Could you check a few things on this drawing? It's one solid part, dimensions in mm from its lowest x, y, z. A direction names the side the tool comes from. Give positions to 0.01 mm unless a question says otherwise; leave off trailing zeros. Loops run counter-clockwise (first coordinate to the right, second up) from the corner with the lowest first, then second, coordinate; pieces in that order, holes last. Notation, with made-up numbers: M 25.5,61 L 70.5,61 A38 ccw 70.5,99 Z; hole C 74,87.5 d9. An arc over 180 degrees is marked long. One line per item, written item: value. Start each with the question number.
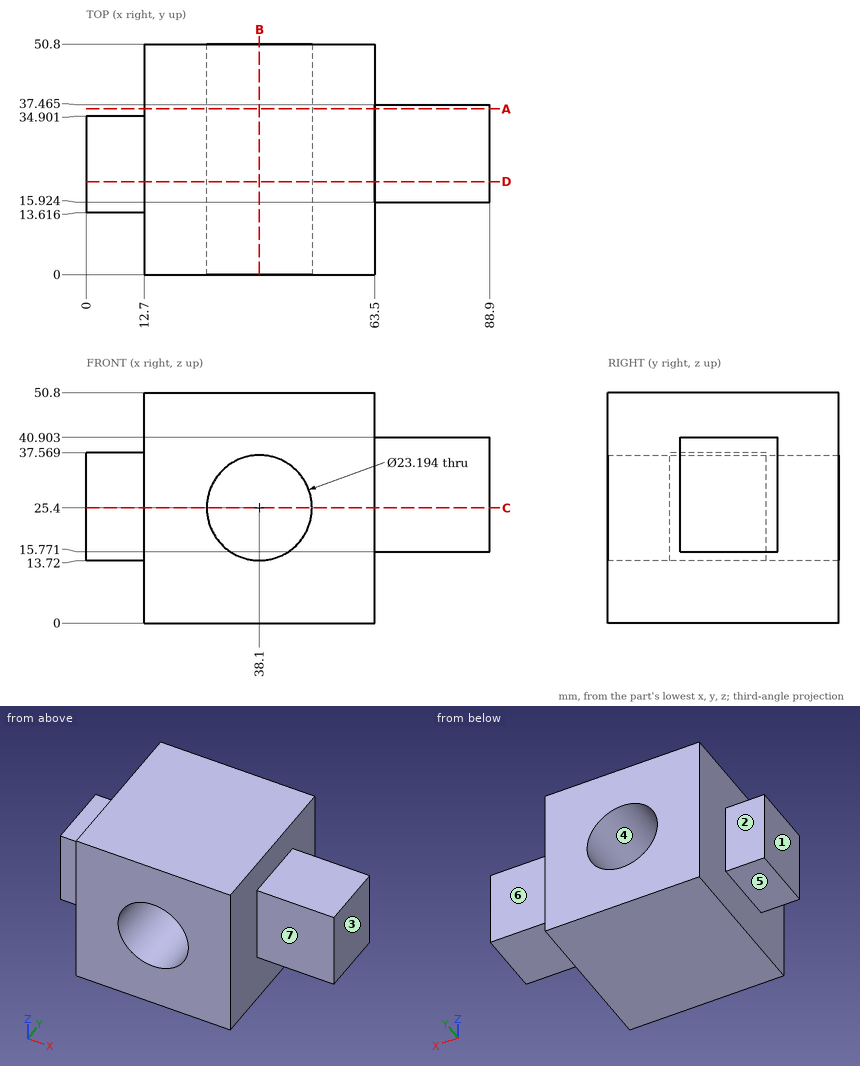
Q1. If we section it at A-A, the plane y = 36.5: Write out the boundary of the cut face in (x, z).
Q2. If we mould it in two halves opening along X, with no side actions, what happens to the marked faces 1, 2, 3 and 4? For each: released by +X, released by -X, zero draft, split by the parting line, or undercut.
Q3. Which directions (+Z, -Z, +X, -X, +Y, -Y) give clear straight access to the entire face, cutting with the end or side of a thin tool? Please do the marked faces 5, 6 and 7.
Q4. If we section it at B-B, the plane x = 38.1: Write out the boundary of the cut face in (y, z).
Q5. For P1, Ø4, axis at y = 23.5, z = 23.5, coming from the -X side; P2, Ø1, axis at y = 35.5, z = 16.5, coming from the -X side; P3, Ø6.5, axis at x = 70, y = 28.5, coming from the -Z side; P4, Ø6.5, axis at x = 8, z = 21, coming from the +Y side, each with a flat end and sliding along its axis, tell me the tip position at first contact or that it passes through.
Q6. If we section it at C-C, the plane z = 25.4: Write out the boundary of the cut face in (x, y) (1 decimal).
Q7. I need wall thicknesses on line 1 along Z through (x, y) = (38, 14); line 2 along X through (y, z) = (15, 25); line 3 along X through (y, z) = (29, 8). Which ranges of each line are inside material? Lowest first, please.
Q8. If we section it at D-D, the plane y = 20.5: Write out the boundary of the cut face in (x, z).
Response:
1. outline: M 12.7,0 L 63.5,0 L 63.5,15.77 L 88.9,15.77 L 88.9,40.9 L 63.5,40.9 L 63.5,50.8 L 12.7,50.8 Z; hole C 38.1,25.4 d23.19
2. face 1: released by -X
2. face 2: zero draft
2. face 3: released by +X
2. face 4: undercut
3. face 5: -Z, -X, +Y, -Y
3. face 6: +Z, -Z, +X, +Y
3. face 7: +Z, -Z, +X, -Y
4. outline: M 0,0 L 50.8,0 L 50.8,13.8 L 0,13.8 Z; M 0,37 L 50.8,37 L 50.8,50.8 L 0,50.8 Z
5. P1: x = 0
5. P2: x = 12.7
5. P3: z = 15.77
5. P4: y = 34.9
6. outline: M 0,13.6 L 12.7,13.6 L 12.7,0 L 26.5,0 L 26.5,50.8 L 12.7,50.8 L 12.7,34.9 L 0,34.9 Z; M 49.7,0 L 63.5,0 L 63.5,15.9 L 88.9,15.9 L 88.9,37.5 L 63.5,37.5 L 63.5,50.8 L 49.7,50.8 Z
7. line 1: 0 to 13.8, 37 to 50.8
7. line 2: 0 to 26.51, 49.69 to 63.5
7. line 3: 12.7 to 63.5
8. outline: M 0,13.72 L 12.7,13.72 L 12.7,0 L 63.5,0 L 63.5,15.77 L 88.9,15.77 L 88.9,40.9 L 63.5,40.9 L 63.5,50.8 L 12.7,50.8 L 12.7,37.57 L 0,37.57 Z; hole C 38.1,25.4 d23.19
